from build123d import *

# Parameters (mm, degrees)
EXTRUDE_1_DEPTH     = 2
SKETCH_2_R          = 1.1
SKETCH_2_R_2        = 2.55
CUT_EXTRUDE_1_DEPTH = 29.354893758


with BuildPart() as part:
    # 草图1 → 凸台-拉伸1 (new body)
    with BuildSketch(Plane(origin=(0, 0, 0), x_dir=(0, 0, -1), z_dir=(1, 0, 0))):
        with BuildLine():
            Line((20, 0), (0, 0))
            Line((0, 0), (0, -20))
            Line((0, -20), (8.25, -20))
            ThreePointArc((8.25, -20), (10, -18.25), (11.75, -20))
            Line((11.75, -20), (20, -20))
            Line((20, -20), (20, 0))
        make_face()
    extrude(amount=EXTRUDE_1_DEPTH)

    # 草图2 → 切除-拉伸1 (cut, through all)
    with BuildSketch(Plane(origin=(2, 0, 0), x_dir=(0, 0, -1), z_dir=(1, 0, 0))):
        with Locations((15.656854249, -18)):
            Circle(SKETCH_2_R)
        with Locations((13.815658986, -12.5)):
            Circle(SKETCH_2_R_2)
    extrude(amount=-CUT_EXTRUDE_1_DEPTH, mode=Mode.SUBTRACT)


solid = part.part
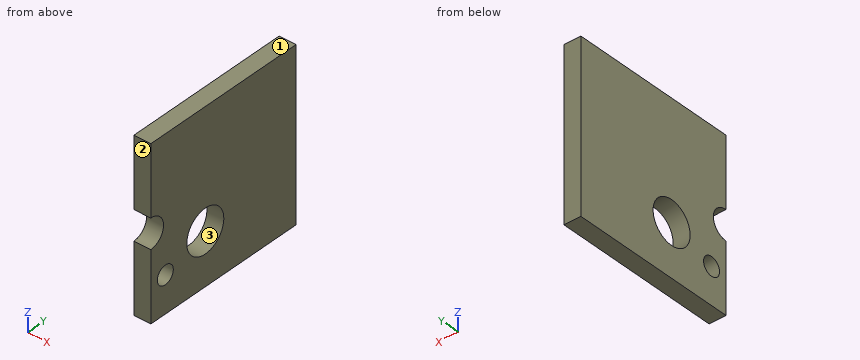
Input: part model. Units: mm. Frame: model coordinates. Face numbers are marked on the shaded views. Coordinates: 2 decimals unless noted, no trailing zeros. Loops run counter-clockwise (first coordinate to the right, second up) from the corner with the lowest first, then second, coordinate; pieces in that order, holes last.
Q1. Draft query along Z for the marked faces 1, 2 and 3. Return one class per face: +Z half, -Z half, draft (parallel to the pull), parting line (faces both ways), or undercut.
Q2. Cut plane A-A (y = -12.5). Output: boundary loops of the cut face in (x, z), then the cut area to 3 significant figures.
Q3. Cut plane D-D (z = -10). Output: boundary loops of the cut face in (x, y), then the cut area to 3 significant figures.
Q4. Cut plane C-C (y = -18). Output: boundary loops of the cut face in (x, z), then the cut area to 3 significant figures.
Q5. Contact query for a flat-ended pin moving along its axis: pin 1 (3 mm diameter, centred on y = -12.5, z = -13.82, fed in from +X). Output: stop coordinate, or through.
Q6. Material intervals for line 1 (Y direction, x = 0.1, z = -8.5); line 2 (Y direction, x = 1.85, z = -16); line 3 (Y direction, x = 1.45, z = -13.25), sorted ascending.
Q7. Cut plane B-B (x = 1.5). Output: boundary loops of the cut face in (y, z).
Working result:
1. face 1: +Z half
1. face 2: draft
1. face 3: undercut
2. outline: (0, -20) - (2, -20) - (2, -16.37) - (0, -16.37) - close; (0, -11.27) - (2, -11.27) - (2, 0) - (0, 0) - close
2. area: 29.8 mm2
3. outline: (0, -18.25) - (2, -18.25) - (2, 0) - (0, 0) - close
3. area: 36.5 mm2
4. outline: (0, -20) - (2, -20) - (2, -16.76) - (0, -16.76) - close; (0, -14.56) - (2, -14.56) - (2, 0) - (0, 0) - close
4. area: 35.6 mm2
5. pin 1: passes through
6. line 1: y = -19.1 to 0
6. line 2: y = -20 to -19.05, -16.95 to -13.82, -11.18 to 0
6. line 3: y = -20 to -14.99, -10.01 to 0
7. outline: (-20, -20) - (0, -20) - (0, 0) - (-20, 0) - (-20, -8.25) arc R1.75 cw to (-20, -11.75) - close; hole circle Ø2.2 at (-18, -15.66); hole circle Ø5.1 at (-12.5, -13.82)
